from build123d import *

# Parameters (mm, degrees)
F1_DEPTH = 3
F3_D     = 10
F3_DEPTH = 9
F3_TIP   = 3.0043030951
F4_SIZE  = 2.99999


# Not quite as in the source:
# - a fillet or chamfer is up to 0.001 mm smaller than in the source, because OpenCascade refuses the exact size


with BuildPart() as f1:
    # F0 (on Front) → F1 (new body)
    with BuildSketch(Plane.XZ):
        with BuildLine():
            Line((0, 45), (0, 0))
            Line((0, 0), (135, 0))
            Line((135, 0), (135, 45))
            ThreePointArc((135, 45), (103.1801948466, 58.1801948466), (90, 90))
            Line((90, 90), (45, 90))
            ThreePointArc((45, 90), (31.8198051534, 58.1801948466), (0, 45))
        make_face()
    extrude(amount=F1_DEPTH)

    # F3
    with Locations(Plane.XZ.offset(3)):
        with Locations((57, 78), (78, 78), (123, 33), (123, 12), (12, 12), (12, 33)):
            Hole(F3_D / 2, depth=F3_DEPTH)
            with Locations((0, 0, -(F3_DEPTH + F3_TIP / 2))):  # 118° drill point
                Cone(0, F3_D / 2, F3_TIP, mode=Mode.SUBTRACT)

    # F4 (size 3 in the source; OpenCascade refuses exactly that, so slightly less here)
    f4_edges = [f1.edges().sort_by_distance(p)[0] for p in [
        (31.819805, -3, 58.180195),
        (67.5, -3, 90),
        (103.180195, -3, 58.180195),
        (135, -3, 22.5),
        (0, -3, 22.5),
        (67.5, -3, 0),
    ]]
    chamfer(f4_edges, length=F4_SIZE)


solid = f1.part
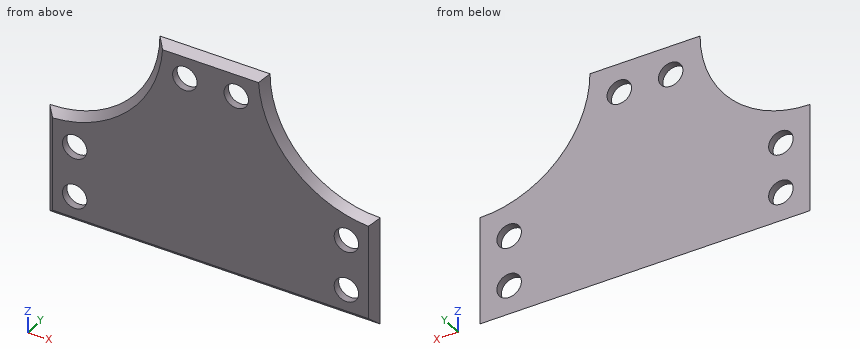
Read the model definition and answer for the solid it produces. Units are mm, in the model's axes. Round coordinates to 2 decimals unless told otherwise and drop trailing zeros. Order: outer loops, then holes, each group sorted by start corner. A loop starts at its lowest first (then second) coordinate and runs counter-clockwise, first axis right, second up.
1) A flat-ended cylindrical pin translates along its axis: pin 1 (1 mm diameter, centred on y = -1.5, z = 69, fed in from +X). Find the tip coordinate at first contact, or state that the pin passes through.
2) Straight lines are drawn through the part: L1, parallel to X at y = -0.5, z = 7.5; L2, parallel to X at y = -1.5, z = 8; L3, parallel to Z at x = 123, y = -1.7. For each, find the intervals that lie inside material, in ascending order.
3) The part is cut by section C-C on y = -1. Write down the section's boundary in (x, z), plus the area to 3 significant figures.
4) The part is cut by section B-B on z = 15. Give the number of separate pieces and of enclosed holes in the cut face, plus the area to 3 significant figures.
Resolved:
1. pin 1: stops at x = 94.13
2. L1: x = 0.5 to 9.82, 14.18 to 120.82, 125.18 to 134.5
2. L2: x = 1.5 to 9, 15 to 120, 126 to 133.5
2. L3: z = 1.7 to 7, 17 to 28, 38 to 44.87
3. outline: (1, 1) - (134, 1) - (134, 44.01) arc R46 cw to (89.01, 89) - (45.99, 89) arc R46 cw to (1, 44.01) - close; hole circle Ø10 at (12, 12); hole circle Ø10 at (12, 33); hole circle Ø10 at (57, 78); hole circle Ø10 at (78, 78); hole circle Ø10 at (123, 12); hole circle Ø10 at (123, 33)
3. area: 8,090 mm2
4. separate pieces: 3
4. enclosed holes: 0
4. area: 348 mm2
